Design review of the part built by this model. Coordinates are the model's own, in mm. A direction names the side the tool comes from. Coordinates: 2 decimals unless noted, no trailing zeros. Loops run counter-clockwise (first coordinate to the right, second up) from the corner with the lowest first, then second, coordinate; pieces in that order, holes last. Notation, with made-up numbers: (2, 62.25) -> (50, 62.25) arc R6 ccw to (50, 66.25) -> close; hole circle Ø5 at (-31.5, 41.5). An arc over 180 degrees is marked (long way). Use a Markdown table: item, result. Add a question column.
Q1. For faces 5 (the face through (81.33, -21.84, 8.63)), 6 (the face through (-115, 37, 4)), 7 (the face through (-67.38, 14.76, 1.48)), list the 3-axis set-ups (+Z, -Z, +X, -X, +Y, -Y) from which the entire face can be reached by the end or side of a thin tool; tool diameter is ignored.
Q2. Draft analysis for pull direction Y (two halves, no side actions). For faces 1 (the face through (-105, 19, 33)), 2 (the face through (-105.728, 21.707, 8.63)), 3 (the face through (-70.691, -9.926, 1.479)), 4 (the face through (1.3, -71.06, 1.48)), state which applies: pulls with the +Y half, pulls with the -Y half, needs draft (parallel to the pull), parting line crosses it, or undercut.
Q3. Take a section at D-D on y = 119. Write out the cut boundary in (x, z), plus the area to 3 significant figures.
Q4. Take a section at B-B on x = 93.5. Write out the cut boundary in (y, z).
Q5. Clearance check with flat-ended pins moving along their axes: pin 1 Ø17.5 at (x, y) = (50, 174) entering from +Z; pin 2 Ø6.5 at (y, z) = (186.61, 14.63) entering from +X; pin 3 Ø10 at (x, z) = (-142, 3.5) entering from -Y; pin 4 Ø13.5 at (x, y) = (-114.5, 21.5) entering from -Z. State where each tip first meets the part, or that it passes through.
Q6. Take a section at A-A on x = -66. Write out the cut boundary in (y, z).
Q7. Take a section at C-C on x = -113.5. Write out the cut boundary in (y, z), plus the area to 3 significant figures.
Q8. For probe 1 along X at (y, z) = (22.5, 2); probe 2 along Z at (x, y) = (15.5, -133); probe 3 along Y at (x, z) = (-93.5, 0.95), list the stretches that pass through material, from the lowest coordinate up.
from build123d import *

# Parameters (mm, degrees)
BOSS_EXTRUDE1_DEPTH = 3
CUT_EXTRUDE2_DEPTH  = 10
CUT_EXTRUDE3_DEPTH  = 10
BOSS_EXTRUDE2_DEPTH = 4
SKETCH6_W           = 5
SKETCH6_H           = 54
BOSS_EXTRUDE3_DEPTH = 30
SKETCH8_R           = 2
SKETCH8_W           = 40
SKETCH8_H           = 20
CUT_EXTRUDE4_DEPTH  = 40
SKETCH9_R           = 2
SKETCH9_W           = 40
SKETCH9_H           = 20
CUT_EXTRUDE5_DEPTH  = 40
SKETCH13_R          = 2.5
SKETCH13_W          = 20
SKETCH13_H          = 40
CUT_EXTRUDE6_DEPTH  = 40
SKETCH14_R          = 10
CUT_EXTRUDE7_DEPTH  = 10


with BuildPart() as part:
    # Sketch2 → Boss-Extrude1 (new body)
    with BuildSketch(Plane.XY):
        Polygon((-187, 161.946750508), (187, 161.946750508), (0, -161.946750508), align=None)
    extrude(amount=BOSS_EXTRUDE1_DEPTH)

    # Sketch3 → Cut-Extrude2 (cut)
    with BuildSketch(Plane.XY):
        Polygon((-83.5, -17.320508076), (-57.519237886, -2.320508076), (-77.519237886, 32.320508076), (-103.5, 17.320508076), align=None)
        Polygon((57.519237886, -2.320508076), (83.5, -17.320508076), (103.5, 17.320508076), (77.519237886, 32.320508076), align=None)
    extrude(amount=CUT_EXTRUDE2_DEPTH, mode=Mode.SUBTRACT)

    # Sketch4 → Cut-Extrude3 (cut)
    with BuildSketch(Plane.XY):
        Polygon((0, 131.946750508), (20, 131.946750508), (20, 161.946750508), (0, 161.946750508), (-20, 161.946750508), (-20, 131.946750508), align=None)
    extrude(amount=CUT_EXTRUDE3_DEPTH, mode=Mode.SUBTRACT)

    # Sketch5 → Boss-Extrude2 (add)
    with BuildSketch(Plane.XY):
        Polygon((-103.5, 17.320508076), (-80.25426683, 30.543976819), (-100.117314098, 65.461524227), (-123.5, 51.961524227), (-146.882685902, 38.461524227), (-126.882685902, 3.820508076), align=None)
        Polygon((20, 161.946750508), (20, 134.946750508), (60, 134.946750508), (60, 161.946750508), (60, 188.946750508), (20, 188.946750508), align=None)
        Polygon((83.5, -17.320508076), (60.117314098, -3.820508076), (40.117314098, -38.461524227), (63.5, -51.961524227), (86.882685902, -65.461524227), (106.882685902, -30.820508076), align=None)
    extrude(amount=BOSS_EXTRUDE2_DEPTH)

    # Sketch6 → Boss-Extrude3 (add)
    with BuildSketch(Plane.XY.offset(3)):
        Polygon((-126.882685902, 3.820508076), (-80.25426683, 30.543976819), (-82.726527648, 34.89000103), (-129.382685902, 8.150635095), align=None)
        Polygon((60.117314098, -3.820508076), (106.882685902, -30.820508076), (104.382685902, -35.150635095), (57.617314098, -8.150635095), align=None)
        with Locations((22.5, 161.946750508)):
            Rectangle(SKETCH6_W, SKETCH6_H)
    extrude(amount=BOSS_EXTRUDE3_DEPTH)

    # Sketch8 → Cut-Extrude4 (cut)
    with BuildSketch(Plane(origin=(-33.019892419, 57.614727947, 0), x_dir=(0.867611975, 0.497241853, 0), z_dir=(0.497241853, -0.867611975, 0))):
        with Locations((-56.728666482, 15.70430261)):
            Circle(SKETCH8_R)
        with Locations((-56.728666482, 25.70430261)):
            Circle(SKETCH8_R)
        with Locations((-105.728666482, 25.70430261)):
            Circle(SKETCH8_R)
        with Locations((-105.728666482, 15.70430261)):
            Circle(SKETCH8_R)
        with Locations((-81.228666482, 20.70430261)):
            Rectangle(SKETCH8_W, SKETCH8_H)
    extrude(amount=-CUT_EXTRUDE4_DEPTH, mode=Mode.SUBTRACT)

    # Sketch9 → Cut-Extrude5 (cut)
    with BuildSketch(Plane(origin=(10.875, 18.836052532, 0), x_dir=(0.866025404, -0.5, 0), z_dir=(-0.5, -0.866025404, 0))):
        with Locations((105.471828454, 15.12829127)):
            Circle(SKETCH9_R)
        with Locations((105.471828454, 25.12829127)):
            Circle(SKETCH9_R)
        with Locations((56.471828454, 25.12829127)):
            Circle(SKETCH9_R)
        with Locations((56.471828454, 15.12829127)):
            Circle(SKETCH9_R)
        with Locations((80.971828454, 20.12829127)):
            Rectangle(SKETCH9_W, SKETCH9_H)
    extrude(amount=-CUT_EXTRUDE5_DEPTH, mode=Mode.SUBTRACT)

    # Sketch13 → Cut-Extrude6 (cut)
    with BuildSketch(Plane(origin=(25, 0, 0), x_dir=(0, 0, -1), z_dir=(1, 0, 0))):
        with Locations((-26.890806587, 137.608868151)):
            Circle(SKETCH13_R)
        with Locations((-14.632269725, 137.608868151)):
            Circle(SKETCH13_R)
        with Locations((-26.890806587, 186.608868151)):
            Circle(SKETCH13_R)
        with Locations((-14.632269725, 186.608868151)):
            Circle(SKETCH13_R)
        with Locations((-19.755862456, 162.108868151)):
            Rectangle(SKETCH13_W, SKETCH13_H)
    extrude(amount=-CUT_EXTRUDE6_DEPTH, mode=Mode.SUBTRACT)

    # Sketch14 → Cut-Extrude7 (cut)
    with BuildSketch(Plane(origin=(0, 0, 0), x_dir=(-1, 0, 0), z_dir=(0, 0, -1))):
        with Locations((0, -80.973375254)):
            Circle(SKETCH14_R)
        with Locations((93.5, 80.973375254)):
            Circle(SKETCH14_R)
        with Locations((-93.5, 80.973375254)):
            Circle(SKETCH14_R)
    extrude(amount=-CUT_EXTRUDE7_DEPTH, mode=Mode.SUBTRACT)


solid = part.part
Answer list:
| question | item | result |
|---|---|---|
| 1 | face 5 | +Z, -X, -Y |
| 1 | face 6 | +Z, -X, +Y |
| 1 | face 7 | +Z, -Z |
| 2 | face 1 | needs draft |
| 2 | face 2 | pulls with the +Y half |
| 2 | face 3 | undercut |
| 2 | face 4 | undercut |
| 3 | outline | (-162.2, 0) -> (162.2, 0) -> (162.2, 3) -> (-162.2, 3) -> close |
| 3 | area | 973 mm² |
| 4 | outline | (-54, 0) -> (-23.09, 0) -> (-23.09, 10.13) -> (-28.87, 10.13) -> (-28.87, 4) -> (-54, 4) -> close; (-28.87, 30.13) -> (-23.09, 30.13) -> (-23.09, 33) -> (-28.87, 33) -> close; (23.09, 0) -> (70.97, 0) -> (70.97, 3) -> (23.09, 3) -> close; (90.97, 0) -> (161.95, 0) -> (161.95, 3) -> (90.97, 3) -> close |
| 5 | pin 1 | z = 4 |
| 5 | pin 2 | x = 25 |
| 5 | pin 3 | y = 21.34 |
| 5 | pin 4 | z = 0 |
| 6 | outline | (-47.63, 0) -> (-7.22, 0) -> (-7.22, 3) -> (-47.63, 3) -> close; (12.37, 0) -> (161.95, 0) -> (161.95, 3) -> (12.37, 3) -> close |
| 7 | outline | (11.49, 3) -> (11.55, 3) -> (11.55, 0) -> (161.95, 0) -> (161.95, 3) -> (57.74, 3) -> (57.74, 4) -> (17.25, 4) -> (17.25, 10.7) -> (11.49, 10.7) -> close; (11.49, 30.7) -> (17.25, 30.7) -> (17.25, 33) -> (11.49, 33) -> close |
| 7 | area | 549 mm² |
| 8 | probe 1 | -137.67 to -94.39, -71.85 to 71.85, 94.53 to 106.49 |
| 8 | probe 2 | 0 to 3 |
| 8 | probe 3 | 23.01 to 70.97, 90.97 to 161.95 |
